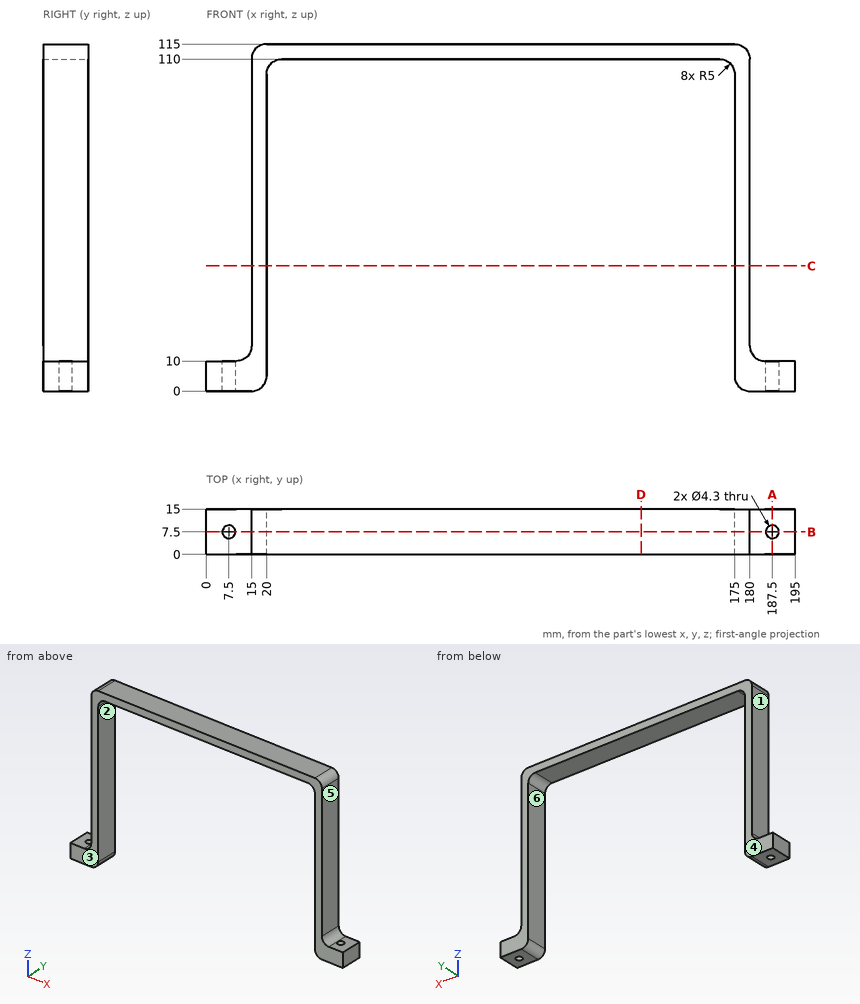
Source: three-view drawing plus pictorial views. Frame: mm from the lowest corner of the part. A direction names the side the tool comes from. Give positions to 0.01 mm unless a question says otherwise; leave off trailing zeros. Loops run counter-clockwise (first coordinate to the right, second up) from the corner with the lowest first, then second, coordinate; pieces in that order, holes last. Notation, with made-up numbers: (-31, 28.25) -> (28, 28.25) arc R30 ccw to (28, 57.25) -> close; hole circle Ø10 at (54, 89). An arc over 180 degrees is marked (long way). Use a Markdown table: item, result. Add a question column.
(1) Ray query, line 1 (X direction, y = 7.5, z = 24); line 2 (X direction, y = 5.25, z = 9.5); line 3 (Z direction, x = 163.5, y = 12). Return the intervals inside material, ascending.
(2) First-contact query: pin 1 Ø5 at (y, z) = (3.5, 65.5) entering from +X; pin 2 Ø7.5 at (y, z) = (10.5, 52) entering from -X. Flat tips, straight axial feed; report the tip coordinate or a pass-through.
(3) Section query C-C (z = 41.5). Output: boundary loops of the cut face in (x, y), then the cut area to 3 significant figures.
(4) Section query D-D (x = 144). Output: boundary loops of the cut face in (y, z), then the cut area to 3 significant figures.
(5) Access query for the marked faces 4, 5 and 6. Directions: +Z, -Z, +X, -X, +Y, -Y. A direction counts if a zero-diameter tool reaches every point of the face in a straight line with its end or side. Return the directions, or none.
(6) Section query A-A (x = 187.5). Output: boundary loops of the cut face in (y, z), then the cut area to 3 significant figures.
(7) Section query B-B (y = 7.5). Output: boundary loops of the cut face in (x, z), then the cut area to 3 significant figures.
(8) Pull-direction query (X, two-part tool) for the marked faces 1, 2 and 3; classes: +X half, -X half, draft (parallel to the pull), parting line (faces both ways), or undercut.
Checked values:
| question | item | result |
|---|---|---|
| 1 | line 1 | 15 to 20, 175 to 180 |
| 1 | line 2 | 0 to 20, 175 to 195 |
| 1 | line 3 | 110 to 115 |
| 2 | pin 1 | x = 180 |
| 2 | pin 2 | x = 15 |
| 3 | outline | (15, 0) -> (20, 0) -> (20, 15) -> (15, 15) -> close; (175, 0) -> (180, 0) -> (180, 15) -> (175, 15) -> close |
| 3 | area | 150 mm^2 |
| 4 | outline | (0, 110) -> (15, 110) -> (15, 115) -> (0, 115) -> close |
| 4 | area | 75.0 mm^2 |
| 5 | face 4 | +Z, -Z, +X, -X, +Y |
| 5 | face 5 | +Z, +X, +Y, -Y |
| 5 | face 6 | -Z, +Y, -Y |
| 6 | outline | (0, 0) -> (5.35, 0) -> (5.35, 10) -> (0, 10) -> close; (9.65, 0) -> (15, 0) -> (15, 10) -> (9.65, 10) -> close |
| 6 | area | 107 mm^2 |
| 7 | outline | (0, 0) -> (5.35, 0) -> (5.35, 10) -> (0, 10) -> close; (9.65, 0) -> (15, 0) arc R5 ccw to (20, 5) -> (20, 105) arc R5 cw to (25, 110) -> (170, 110) arc R5 cw to (175, 105) -> (175, 5) arc R5 ccw to (180, 0) -> (185.35, 0) -> (185.35, 10) -> (185, 10) arc R5 cw to (180, 15) -> (180, 110) arc R5 ccw to (175, 115) -> (20, 115) arc R5 ccw to (15, 110) -> (15, 15) arc R5 cw to (10, 10) -> (9.65, 10) -> close; (189.65, 0) -> (195, 0) -> (195, 10) -> (189.65, 10) -> close |
| 7 | area | 2,140 mm^2 |
| 8 | face 1 | -X half |
| 8 | face 2 | undercut |
| 8 | face 3 | draft |
